Autodesk Inventor part; units mm, degrees
ref_plane "Work Plane1" through (9.2, 14.95, 24.1) normal (0, 0, -1) x (1, 0, 0)
ref_plane "YZ Plane" through (0, 0, 0) normal (1, 0, 0) x (0, 1, 0)
ref_plane "XZ Plane" through (0, 0, 0) normal (0, 1, 0) x (-1, 0, 0)
sketch "Sketch1" plane through (0, 0, 0) normal (1, 0, 0) x (0, 1, 0)
  line L0 (20, 20.4) -> (0, 20.4)
  line L1 (0, 20.4) -> (0, -20.4)
  line L2 (0, -20.4) -> (20, -20.4)
  line L3 (20, -20.4) -> (20, 20.4)
  line L4 (0, -28.56) -> (0, 28.56)
  line L5 (-4, 0) -> (24, 0)
  point P0 (0, 0)
  dimension "d0" = 40.8
  dimension "d1" = 20
extrude "Extrusion1" add sketch "Sketch1" along normal blind 38.4
sketch "Sketch2" plane through (0, 0, 0) normal (1, 0, 0) x (0, 1, 0)
  line L0 (20, 20.4) -> (0, 20.4)
  line L1 (20, -20.4) -> (20, 20.4)
  line L2 (0, -20.4) -> (20, -20.4)
  line L3 (0, 20.4) -> (0, -20.4)
  line L4 (10, 20.4) -> (10, -20.4)
  line L5 (0, 20.4) -> (0, -20.4)
  circle A0 centre (10, 10.35) radius 2.95
  point P0 (0, 0)
  dimension "d4" = 5.9
  dimension "d40" = 10.05
extrude "Extrusion2" add sketch "Sketch2" against normal blind 3.5 contours A0 L4 | L4 A0
sketch "Sketch3" plane through (0, 0, 20.4) normal (0, 0, 1) x (1, 0, 0)
  line L0 (9.2, 20) -> (11.7, 20)
  line L1 (11.7, 20) -> (11.7, 0)
  line L2 (11.7, 0) -> (9.2, 0)
  line L3 (9.2, 0) -> (9.2, 20)
  line L4 (0, 20) -> (0, 0)
  line L5 (0, 0) -> (38.4, 0)
  line L6 (38.4, 20) -> (38.4, 0)
  line L7 (0, 20) -> (38.4, 20)
  point P0 (0, 0)
  dimension "d7" = 2.5
  dimension "d9" = 9.2
  dimension "d10" = 26.7
extrude "Extrusion3" add sketch "Sketch3" along normal blind 6.55 contours L0 L1 L2 L3
sketch "Sketch4" plane through (0, 0, -20.4) normal (0, 0, -1) x (-1, 0, 0)
  line L0 (-11.7, 20) -> (-9.2, 20)
  line L1 (-9.2, 20) -> (-9.2, 0)
  line L2 (-9.2, 0) -> (-11.7, 0)
  line L3 (-11.7, 0) -> (-11.7, 20)
  line L4 (0, 0) -> (0, 20)
  line L5 (0, 20) -> (-38.4, 20)
  line L6 (-38.4, 0) -> (-38.4, 20)
  line L7 (0, 0) -> (-38.4, 0)
  point P0 (0, 0)
  dimension "d13" = 2.5
  dimension "d14" = 9.2
  dimension "d15" = 26.7
extrude "Extrusion4" add sketch "Sketch4" along normal blind 6.55 contours L0 L1 L2 L3
sketch "Sketch5" plane through (9.2, 0, 20.4) normal (-1, 0, 0) x (0, 0, 1)
  circle A0 centre (-10.05, 10) radius 2.95
  line L0 (0, 20) -> (0, 0)
  line L1 (-40.8, 20) -> (0, 20)
  line L2 (-40.8, 0) -> (-40.8, 20)
  line L3 (0, 0) -> (-40.8, 0)
  line L4 (0, 20) -> (0, 0)
  line L5 (0, 20) -> (6.55, 20)
  line L6 (6.55, 0) -> (6.55, 20)
  line L7 (0, 0) -> (6.55, 0)
  line L8 (-40.8, 0) -> (-40.8, 20)
  line L9 (-40.8, 0) -> (-47.35, 0)
  line L10 (-47.35, 20) -> (-47.35, 0)
  line L11 (-40.8, 20) -> (-47.35, 20)
  circle A1 centre (3.7, 14.95) radius 2.2
  arc A2 (5.3971, 6.45) -> (5.3971, 3.65) centre (3.7, 5.05) ccw
  circle A3 centre (-44.5, 14.95) radius 2.2
  circle A4 centre (-44.5, 5.05) radius 2.2
  line L12 (-47.35, 10) -> (6.55, 10) construction
  line L13 (-20.4, 0) -> (-20.4, 20) construction
  line L14 (6.55, 6.45) -> (5.3971, 6.45)
  line L15 (5.3971, 3.65) -> (6.55, 3.65)
  line L16 (6.55, 3.65) -> (6.55, 6.45)
  line L17 (3.7, 5.05) -> (6.55, 5.05) construction
  line L18 (3.7, 5.05) -> (3.7, 20) construction
  line L19 (-44.5, 5.05) -> (6.55, 5.05) construction
  point P0 (6.55, 3.65)
  point P1 (6.55, 6.45)
  dimension "d18" = 4.4
  dimension "d19" = 4.4
  dimension "d20" = 4.4
  dimension "d21" = 4.4
  dimension "d22" = 48.2
  dimension "d23" = 48.2
  dimension "d24" = 9.9
  dimension "d25" = 9.9
  dimension "d26" = 24.1
  dimension "d27" = 4.95
  dimension "d28" = 2.8
extrude "Extrusion5" cut sketch "Sketch5" against normal blind 6.55 contours L6 L15 A2 L14 | A1 | A3 | A4
ref_plane "Work Plane1" through (9.2, 14.95, 24.1) normal (0, 0, -1) x (1, 0, 0)
sketch "Sketch6" plane through (9.2, 14.95, 24.1) normal (0, 0, -1) x (1, 0, 0)
  line L0 (2.5, 2.2) -> (2.5, -2.2)
  line L1 (0, -2.2) -> (0, 2.2)
  line L2 (-21.08, 0) -> (37.58, 0)
  line L3 (0, -2.2) -> (2.5, -2.2)
  line L4 (0, 2.2) -> (2.5, 2.2)
  line L5 (0, 1.4) -> (2.5, 1.4)
  line L6 (2.5, 1.4) -> (2.5, -1.4)
  line L7 (2.5, -1.4) -> (0, -1.4)
  line L8 (0, -1.4) -> (0, 1.4)
  point P0 (-9.2, 14.95)
  point P1 (0, -1.4)
  point P2 (2.5, -1.4)
  point P3 (2.5, 1.4)
  point P4 (0, 1.4)
  dimension "d31" = 2.8
extrude "Extrusion6" cut sketch "Sketch6" against normal blind 6.55 contours L0 L2 L1 L5 | L0 L7 L1 L2
sketch "Sketch7" plane through (0, 0, -26.95) normal (0, 0, -1) x (-1, 0, 0)
  line L0 (-12.71, 16.35) -> (-7.7221, 16.35)
  line L1 (-7.7221, 16.35) -> (-7.7221, 13.55)
  line L2 (-7.7221, 13.55) -> (-12.71, 13.55)
  line L3 (-12.71, 13.55) -> (-12.71, 16.35)
  line L4 (-13.2403, 6.45) -> (-6.6781, 6.45)
  line L5 (-6.6781, 6.45) -> (-6.6781, 3.65)
  line L6 (-6.6781, 3.65) -> (-13.2403, 3.65)
  line L7 (-13.2403, 3.65) -> (-13.2403, 6.45)
  line L8 (11.88, 14.95) -> (-46.78, 14.95)
  line L9 (11.88, 5.05) -> (-46.78, 5.05)
  point P0 (0, 0)
  dimension "d34" = 2.8
  dimension "d35" = 2.8
extrude "Extrusion7" cut sketch "Sketch7" against normal up to surface contours L0 L1 L8 L3 | L8 L1 L2 L3
extrude "Extrusion8" cut sketch "Sketch7" against normal up to surface contours L4 L5 L9 L7 | L9 L5 L6 L7
properties part number "MG996R"
Input: part model. Units: mm. Frame: model coordinates. A direction names the side the tool comes from. Coordinates: 2 decimals unless noted, no trailing zeros. Loops run counter-clockwise (first coordinate to the right, second up) from the corner with the lowest first, then second, coordinate; pieces in that order, holes last.
Q1. Set-up query: faces 1 (the cylindrical face through (-1.726, 7.053, 10.48)), 2 (the flat face through (10, 16.35, 26)), 3 (the flat face through (9.2, 10, -24)), 4 (the flat face through (11.7, 10, -24)), 5 (the flat face through (10, 16.35, -26)). Return all of +Z, -Z, +X, -X, +Y, -Y with unobstructed straight access to the full face (end or side cutting, diameter ignored); none if empty.
Results are:
face 1: -X
face 2: +Z, +X, -X
face 3: -Z, -X, +Y, -Y
face 4: -Z, +X, +Y, -Y
face 5: -Z, +X, -X
Q2. Contact query for flat-ended pins moving along their axis: pin 1 (2.5 mm diameter, centred on y = 5.05, z = 24.1, fed in from -X); pin 2 (7 mm diameter, centred on y = 11.5, z = -22.5, fed in from -X); pin 3 (12 mm diameter, centred on x = 2, y = 16, fed in from -Z); pin 4 (7.5 mm diameter, centred on x = 3.5, y = 8, fed in from +Z). Output: stop coordinate, or through.
Results are:
pin 1: passes through
pin 2: stops at x = 0
pin 3: stops at z = -20.4
pin 4: stops at z = 20.4
Q3. Section B-B, the plane z = -24.1. Return the cut outline in (x, y), and give its area (3 significant figures).
Results are:
outline: (9.2, 0) - (11.7, 0) - (11.7, 2.85) - (9.2, 2.85) - close; (9.2, 7.25) - (11.7, 7.25) - (11.7, 12.75) - (9.2, 12.75) - close; (9.2, 17.15) - (11.7, 17.15) - (11.7, 20) - (9.2, 20) - close
area: 28.0 mm2
Q4. Section D-D, the plane x = 18.5. Return the cut outline in (y, z).
Results are:
outline: (0, -20.4) - (20, -20.4) - (20, 20.4) - (0, 20.4) - close
Q5. Line query: line 1 along Y through (x, z) = (11.15, -24.1); line 2 along X through (y, z) = (9.25, -19); line 3 along Z through (x, y) = (20, 10.5). Output: solid intervals per line, ascending.
Results are:
line 1: y = 0 to 2.85, 7.25 to 12.75, 17.15 to 20
line 2: x = 0 to 38.4
line 3: z = -20.4 to 20.4
Q6. Mould query, pull axis Y, two halves, no side actions, for faces 6 (the flat face through (19, 0, 0)), 7 (the flat face through (11.7, 10, 24)), 8 (the cylindrical face through (10.4, 15, 21.9)). Classes: +Y half, -Y half, draft (parallel to the pull), parting line (faces both ways), or undercut.
Results are:
face 6: -Y half
face 7: draft
face 8: undercut
Q7. Section C-C, the plane z = 10.35. Return the cut outline in (x, y), and give its area (3 significant figures).
Results are:
outline: (-3.5, 7.05) - (0, 7.05) - (0, 0) - (38.4, 0) - (38.4, 20) - (0, 20) - (0, 12.95) - (-3.5, 12.95) - close
area: 789 mm2
Q8. Section A-A, the plane y = 1.75. Return the cut outline in (x, z), and give its area (3 significant figures).
Results are:
outline: (0, -20.4) - (9.2, -20.4) - (9.2, -26.95) - (11.7, -26.95) - (11.7, -20.4) - (38.4, -20.4) - (38.4, 20.4) - (11.7, 20.4) - (11.7, 26.95) - (9.2, 26.95) - (9.2, 20.4) - (0, 20.4) - close
area: 1,600 mm2
